```python
from build123d import *

# Parameters (mm, degrees)
IZIM2_R                     = 2.5
Y_KSEKLIK_EKSTR_ZYON1_DEPTH = 2.5
DAIRESEL_KAPLAMA1_COUNT     = 3


with BuildPart() as part:
    # izim1 → D_nd_r2 (revolve)
    with BuildSketch(Plane.XY):
        Polygon((0.472431585, 0), (0.472431585, 5), (40.472431585, 5), (44.667929741, 10), (52.967929741, 10), (50.88702434, 0), align=None)
    revolve(axis=Axis((0.472431585, 0, 0), (-1, 0, 0)))



with BuildPart() as body_2:
    # izim2 → D_nd_r3 (revolve)
    with BuildSketch(Plane.XY, mode=Mode.PRIVATE) as d_nd_r3_sk:
        with Locations((55, 31.25)):
            Circle(IZIM2_R)
    revolve(d_nd_r3_sk.sketch.rotate(Axis((0, 0, 0), (1, 0, 0)), 90), axis=Axis((0, 0, 0), (1, 0, 0)))


with BuildPart() as part_1:
    add(part.part)

    add(body_2.part)  # Y_kseklik-Ekstr_zyon1 merges body 2
    # izim3 → Y_kseklik-Ekstr_zyon1 (add, symmetric)
    with BuildSketch(Plane.XY):
        Polygon((51.6, 9.2), (49.564913151, 9.2), (53.984913151, 32.693820177), (56.02, 32.693820177), align=None)
    y_kseklik_ekstr_zyon1 = extrude(amount=Y_KSEKLIK_EKSTR_ZYON1_DEPTH, both=True)

    # Dairesel Kaplama1: Y_kseklik-Ekstr_zyon1 ×3 about axis
    dairesel_kaplama1_axis = Axis((0, 0, 0), (1, 0, 0))
    for i in range(1, DAIRESEL_KAPLAMA1_COUNT):
        add(y_kseklik_ekstr_zyon1.rotate(dairesel_kaplama1_axis, i * 360 / DAIRESEL_KAPLAMA1_COUNT))


solid = part_1.part
```
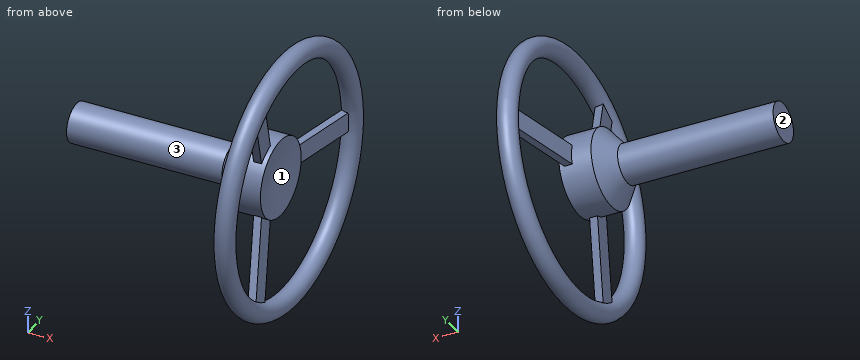
Geometry check sheet. Reference: the model listing, model coordinates, mm. Face numbers are marked on the shaded views. Coordinates: 2 decimals unless noted, no trailing zeros. Order: outer loops, then holes, each group sorted by start corner. A loop starts at its lowest first (then second) coordinate and runs counter-clockwise, first axis right, second up. Notation, with made-up numbers: (-31.75, 27) - (-22.75, 27) arc R14 cw to (-22.75, 35) - close; hole circle Ø1 at (48, -31.5). An arc over 180 degrees is marked (long way). Answer in a Markdown table with one row per item. Add a question column.
1. Material ranges on L1, parallel to Z at x = 44.5, y = 8; L2, parallel to Z at x = 45.5, y = -2.5; L3, parallel to X at y = 25.5, z = 0, recorded low to high. Write a range as [from, to].
2. Gauge pin test, flat ends, axial feed: pin 1 Ø8 at (x, y) = (41, -8) entering from +Z; pin 2 Ø1.5 at (y, z) = (-20, 25.5) entering from -X; pin 3 Ø3 at (x, y) = (33, 1.5) entering from +Z. Record the tip position at first contact, or that the pin passes through.
3. Draft check along Z on the marked faces 1, 2 and 3. Enter one of: +Z half, -Z half, draft (parallel to the pull), parting line (faces both ways), or undercut.
4. Section check A-A (x = 16). Enter the section's corners in (y, z), plus the area to 3 significant figures.
Data:
| question | item | result |
|---|---|---|
| 1 | L1 | z = [-5.66, 5.66] |
| 1 | L2 | z = [-9.68, 9.68] |
| 1 | L3 | x = [52.63, 54.67] |
| 2 | pin 1 | stops at z = 7.7 |
| 2 | pin 2 | stops at x = 52.53 |
| 2 | pin 3 | stops at z = 5 |
| 3 | face 1 | undercut |
| 3 | face 2 | draft |
| 3 | face 3 | parting line |
| 4 | outline | circle Ø10 at (0, 0) |
| 4 | area | 78.5 mm² |
